```python
from build123d import *

# Parameters (mm, degrees)
CHAMFER1_SIZE = 0.5
FILLET1_R     = 1


with BuildPart() as part:
    # Sketch1 → Revolve1 (revolve)
    with BuildSketch(Plane(origin=(0, 0, 0), x_dir=(1, 0, 0), z_dir=(0, 1, 0)), mode=Mode.PRIVATE) as revolve1_sk:
        Polygon((-135, 10), (-135, 0), (135, 0), (135, 8), (135, 10), (102.2, 10), (102.2, 9.5), (100.9, 9.5), (100.9, 10), (29, 10), (29, 12), (-29, 12), (-29, 10), (-100.9, 10), (-100.9, 9.5), (-102.2, 9.5), (-102.2, 10), align=None)
    revolve(revolve1_sk.sketch.rotate(Axis((-135, 0, 0), (1, 0, 0)), 180), axis=Axis((-135, 0, 0), (1, 0, 0)))

    # Chamfer1
    chamfer1_edges = [part.edges().sort_by_distance(p)[0] for p in [
        (-29, 0, -12),
        (29, 0, -12),
    ]]
    chamfer(chamfer1_edges, length=CHAMFER1_SIZE)

    # Fillet1
    fillet1_edges = [part.edges().sort_by_distance(p)[0] for p in [
        (-135, 0, -10),
        (135, 0, -10),
    ]]
    fillet(fillet1_edges, radius=FILLET1_R)


solid = part.part
```
Verification items for the finished model (mm, model axes). A direction names the side the tool comes from. Coordinates: 2 decimals unless noted, no trailing zeros. Write each loop counter-clockwise with the first axis right and the second up, starting at its lowest first coordinate (ties: lowest second). Pieces come first, ordered by that corner, then holes. Notation, with made-up numbers: (-8.5, -23) - (29.5, -23) arc R16 ccw to (29.5, -14) - close; hole circle Ø3 at (24.5, 75). An arc over 180 degrees is marked (long way). One line per question, with ' | ' between items. Start each with the question number.
1. Access from +Z, -Z, +X, -X, +Y, -Y to the whole of each face (thin tool, end or side, straight path). Record for faces 1 (the flat face through (29, -5, 9)), 2 (the flat face through (-102.2, 4, -9)), 3 (the cylindrical face through (-118, 0, -10)).
2. Material ranges on line 1 along Y through (x, z) = (23, 0.5); line 2 along Z through (x, y) = (77, -0.75); line 3 along Y through (x, z) = (-64.5, -1), recorded low to high.
3. Gauge pin test, flat ends, axial feed: P1, Ø5, axis at x = -29, z = 3, coming from the -Y side; P2, Ø1.5, axis at x = 32, z = -2, coming from the -Y side; P3, Ø10, axis at x = -91, y = -1, coming from the -Z side. Record the tip position at first contact, or that the pin passes through.
4. Draft check along X on faces 4 (the cylindrical face through (118, 0, -10)), 5 (the flat face through (135, 0, 0)), 6 (the flat face through (-100.9, 4, 9)). Enter one of: released by +X, released by -X, zero draft, split by the parting line, or undercut.
5. Section check B-B (x = 4). Enter the section's corners in (y, z), plus the area to 3 significant figures.
6. Section check A-A (x = 53). Enter the section's corners in (y, z).
Computed values:
1) face 1: +X | face 2: none | face 3: -X
2) line 1: -11.99 to 11.99 | line 2: -9.97 to 9.97 | line 3: -9.95 to 9.95
3) P1: y = -11.99 | P2: y = -9.92 | P3: z = -10
4) face 4: zero draft | face 5: released by +X | face 6: undercut
5) outline: circle Ø24 at (0, 0) | area: 452 mm²
6) outline: circle Ø20 at (0, 0)
